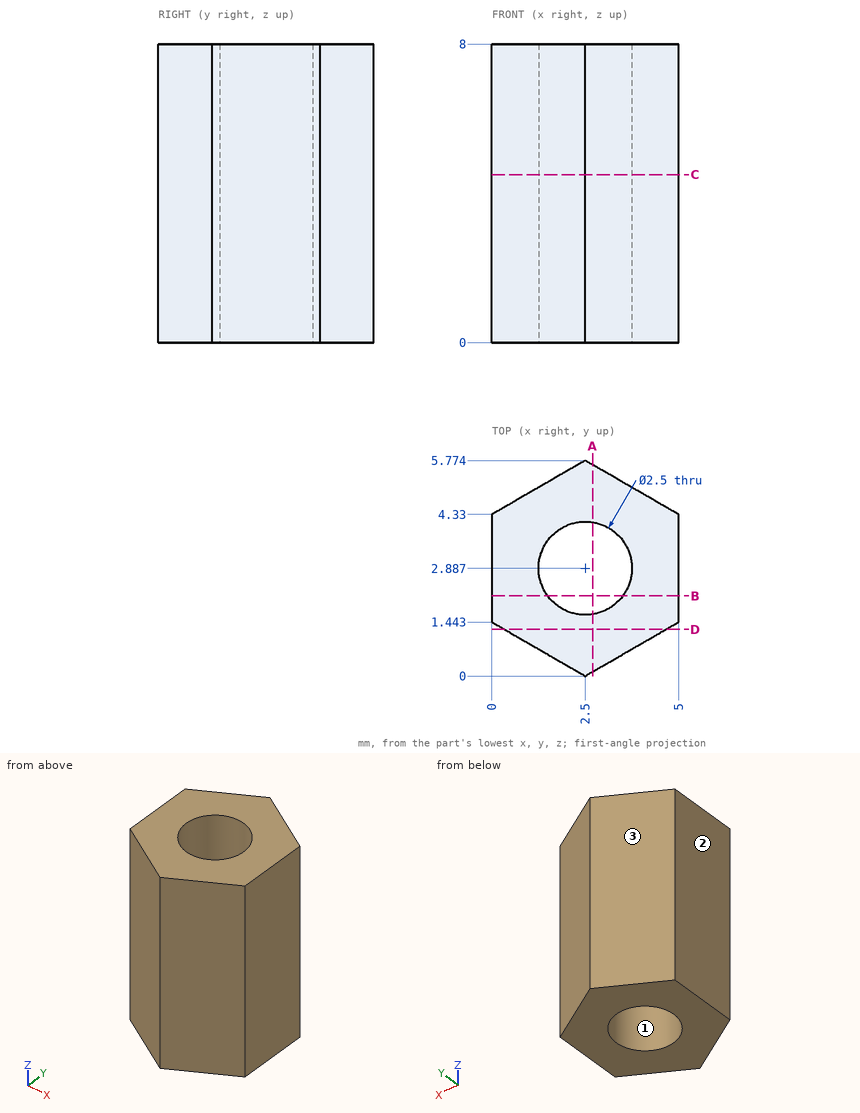
Here's the drawing with two shaded views (mm, measured from the low corner). I have some questions. Round coordinates to 2 decimals unless told otherwise and drop trailing zeros. Loops run counter-clockwise (first coordinate to the right, second up) from the corner with the lowest first, then second, coordinate; pieces in that order, holes last. Notation, with made-up numbers: M -12.75,68.25 L 2.25,68.25 A33 cw 2.25,98.25 Z; hole C -35,-31 d5. An arc over 180 degrees is marked long. Put each result on its own line as item: value.
Q1. Imagine slicing it at B-B (y = 2.15). Write out the boundary of the cut face in (x, z).
Check result:
outline: M 0,0 L 1.49,0 L 1.49,8 L 0,8 Z; M 3.51,0 L 5,0 L 5,8 L 3.51,8 Z
Q2. Thinking about a two-plate mould opening in Y: for the marked faces 1, 2 and 3, which applies, released by +Y, released by -Y, zero draft, split by the parting line, or undercut?
Check result:
face 1: undercut
face 2: zero draft
face 3: released by +Y
Q3. Imagine slicing it at A-A (x = 2.7). Write out the boundary of the cut face in (y, z) (1 decimal).
Check result:
outline: M 0.1,0 L 1.7,0 L 1.7,8 L 0.1,8 Z; M 4.1,0 L 5.7,0 L 5.7,8 L 4.1,8 Z
Q4. I need wall thicknesses on probe 1 along Y at (x, z) = (1.65, 3.5) (1 decimal); probe 2 along Y at (x, z) = (3.1, 5) (1 decimal); probe 3 along X at (y, z) = (2.05, 7.5). Which ranges of each line are inside material? Lowest first, please.
Check result:
probe 1: 0.5 to 2, 3.8 to 5.3
probe 2: 0.3 to 1.8, 4 to 5.4
probe 3: 0 to 1.57, 3.43 to 5
Q5. Imagine slicing it at D-D (y = 1.25). Write out the boundary of the cut face in (x, z) (1 decimal).
Check result:
outline: M 0.3,0 L 4.7,0 L 4.7,8 L 0.3,8 Z
Q6. Imagine slicing it at C-C (z = 4.5). Write out the boundary of the cut face in (x, y).
Check result:
outline: M 0,1.44 L 2.5,0 L 5,1.44 L 5,4.33 L 2.5,5.77 L 0,4.33 Z; hole C 2.5,2.89 d2.5
Q7. For pin 1 (2 mm diameter, centred on x = 2.5, y = 2.89, fed in from -Z), with a flat end and sliding along its axis, tell me the tip position at first contact or that it passes through.
Check result:
pin 1: through
